Work out the finished part from the listing and answer in its coordinate system (mm). A direction names the side the tool comes from. Give positions to 0.01 mm unless a question says otherwise; leave off trailing zeros. Loops run counter-clockwise (first coordinate to the right, second up) from the corner with the lowest first, then second, coordinate; pieces in that order, holes last.
```python
from build123d import *

# Parameters (mm, degrees)
SKETCH1_W           = 76.2
SKETCH1_H           = 44.45
BOSS_EXTRUDE1_DEPTH = 5.08
SKETCH2_R           = 1.5875
BOSS_EXTRUDE6_DEPTH = 6.35
SKETCH3_R           = 1.27
CUT_EXTRUDE1_DEPTH  = 6.35
SKETCH4_W           = 15.24
SKETCH4_H           = 5.08
CUT_EXTRUDE2_DEPTH  = 5.08


with BuildPart() as part:
    # Sketch1 → Boss-Extrude1 (new body)
    with BuildSketch(Plane.XY):
        Rectangle(SKETCH1_W, SKETCH1_H)
    extrude(amount=BOSS_EXTRUDE1_DEPTH)

    # Sketch2 → Boss-Extrude6 (add)
    with BuildSketch(Plane(origin=(0, 0, 0), x_dir=(-1, 0, 0), z_dir=(0, 0, -1))):
        with Locations((0, 4.7625)):
            Circle(SKETCH2_R)
    extrude(amount=-BOSS_EXTRUDE6_DEPTH)

    # Sketch3 → Cut-Extrude1 (cut)
    with BuildSketch(Plane(origin=(0, 0, 0), x_dir=(-1, 0, 0), z_dir=(0, 0, -1))):
        with Locations((4.226013148, -3.773684035)):
            Circle(SKETCH3_R)
        with Locations((-8.536184035, 0.536486852)):
            Circle(SKETCH3_R)
        with Locations((-4.226013147, 13.298684035)):
            Circle(SKETCH3_R)
        with Locations((8.536184035, 8.988513147)):
            Circle(SKETCH3_R)
    extrude(amount=-CUT_EXTRUDE1_DEPTH, mode=Mode.SUBTRACT)

    # Sketch4 → Cut-Extrude2 (cut)
    with BuildSketch(Plane(origin=(0, -22.225, 0), x_dir=(-1, 0, 0), z_dir=(0, -1, 0))):
        with Locations((15.24, -2.54)):
            Rectangle(SKETCH4_W, SKETCH4_H)
        with Locations((-15.24, -2.54)):
            Rectangle(SKETCH4_W, SKETCH4_H)
    extrude(amount=-CUT_EXTRUDE2_DEPTH, mode=Mode.SUBTRACT)


solid = part.part
```
Q1. Which of the six approach directions +Z, -Z, +X, -X, +Y, -Y give full straight-line access (tool end or side, diameter ignored) to faces 5 (the face through (-0.853, 6.101, 5.706)), 6 (the face through (0, 5, 6.35)), 7 (the face through (7.62, -20, 3))?
Q2. Determine the mould class of faces 1 (the face through (4.5, 12.06, 2.5)), 2 (the face through (-8.371, 10.248, 2.504)), 3 (the face through (-1, 22.225, 3)), 4 (the face through (1, 0, 0)) for opening direction Y: +Y half, -Y half, draft (parallel to the pull), parting line (faces both ways), or undercut.
Q3. Section A-A on z = 1.25 is taken. Give the vertices of the cut face in (x, y) (3 decimals), plus the area to 3 significant figures.
Q4. Given pin 1 (5 mm diameter, centred on x = -8.5, y = 1.5, fed in from +Z), flat-ended and moving along its own axis, determine where the tip first touches the part or whether it passes through.
Q5. Section B-B on x = 0 is taken. Give the vertices of the cut face in (y, z) (3 decimals), plus the area to 3 significant figures.
Q6. Consider line 1 along Z through (x, y) = (-16.5, 12); line 2 along Y through (x, z) = (-20.5, 2) (3 decimals); line 3 along Y through (x, z) = (9, 3) (3 decimals). Determine where each line is inside the solid, lowest interval first.
Q7. Section D-D on x = -29 is taken. Give the vertices of the cut face in (y, z) (3 decimals), plus the area to 3 significant figures.
Q8. Section C-C on y = -16 is taken. Give the vertices of the cut face in (x, z).
Check result:
1. face 5: +Z
1. face 6: +Z, +X, -X, +Y, -Y
1. face 7: +Z, -Z, -Y
2. face 1: undercut
2. face 2: undercut
2. face 3: +Y half
2. face 4: draft
3. outline: (-38.1, -22.225) - (-22.86, -22.225) - (-22.86, -17.145) - (-7.62, -17.145) - (-7.62, -22.225) - (7.62, -22.225) - (7.62, -17.145) - (22.86, -17.145) - (22.86, -22.225) - (38.1, -22.225) - (38.1, 22.225) - (-38.1, 22.225) - close; hole circle Ø2.54 at (-8.536, 8.989); hole circle Ø2.54 at (-4.226, -3.774); hole circle Ø2.54 at (4.226, 13.299); hole circle Ø2.54 at (8.536, 0.536)
3. area: 3,210 mm2
4. pin 1: stops at z = 5.08
5. outline: (-22.225, 0) - (22.225, 0) - (22.225, 5.08) - (6.35, 5.08) - (6.35, 6.35) - (3.175, 6.35) - (3.175, 5.08) - (-22.225, 5.08) - close
5. area: 230 mm2
6. line 1: z = 0 to 5.08
6. line 2: y = -17.145 to 22.225
6. line 3: y = -17.145 to -0.646, 1.719 to 22.225
7. outline: (-22.225, 0) - (22.225, 0) - (22.225, 5.08) - (-22.225, 5.08) - close
7. area: 226 mm2
8. outline: (-38.1, 0) - (38.1, 0) - (38.1, 5.08) - (-38.1, 5.08) - close
